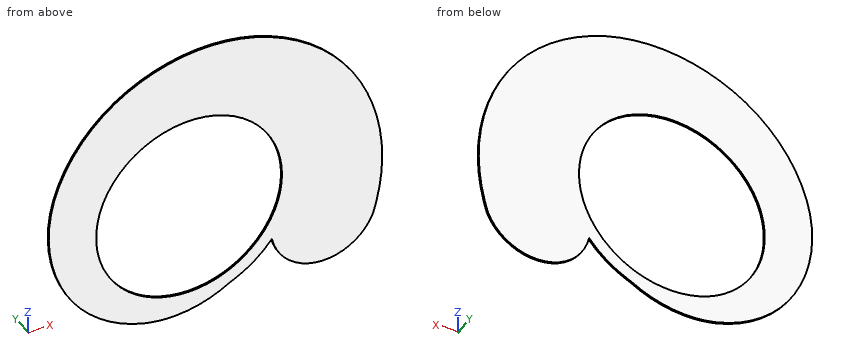
from build123d import *

# Parameters (mm, degrees)
F1_DEPTH = 3.175


with BuildPart() as f1:
    # F0 (on Front) → F1 (new body)
    with BuildSketch(Plane.XZ):
        with BuildLine():
            ThreePointArc((164.2657808805, 68.0411142745), (174.3836228557, 34.6870592545), (177.8, 0))
            ThreePointArc((177.8, 0), (174.3836228557, -34.6870592545), (164.2657808805, -68.0411142745))
            ThreePointArc((164.2657808805, -68.0411142745), (277.9531181005, -7.2739665138), (359.7319413837, -106.9217510028))
            ThreePointArc((359.7319413837, -106.9217510028), (359.3761364248, -115.4172186461), (358.3112136183, -123.8531837399))
            ThreePointArc((358.3112136183, -123.8531837399), (367.281161492, 8.8480312827), (328.531561761, 136.082228549))
            Line((328.531561761, 136.082228549), (164.2657808805, 68.0411142745))
        make_face()
        with BuildLine():
            ThreePointArc((68.0411142745, 164.2657808805), (125.723585695, 125.723585695), (164.2657808805, 68.0411142745))
            Line((164.2657808805, 68.0411142745), (328.531561761, 136.082228549))
            ThreePointArc((328.531561761, 136.082228549), (244.3258111618, 240.7675034736), (126.362069367, 305.0650216352))
            Line((126.362069367, 305.0650216352), (68.0411142745, 164.2657808805))
        make_face()
        with BuildLine():
            ThreePointArc((158.5532229762, -127.0870390081), (157.0041232469, -97.1378663495), (164.2657808805, -68.0411142745))
            ThreePointArc((164.2657808805, -68.0411142745), (137.7338592366, -112.4376450296), (99.5472631467, -147.32))
            ThreePointArc((99.5472631467, -147.32), (93.3013149914, -167.2172179653), (83.1243863135, -185.42))
            ThreePointArc((83.1243863135, -185.42), (124.3088906415, -160.740597571), (158.5532229762, -127.0870390081))
        make_face()
        with BuildLine():
            ThreePointArc((359.7319413837, -106.9217510028), (277.9531181005, -7.2739665138), (164.2657808805, -68.0411142745))
            Line((164.2657808805, -68.0411142745), (258.1319413837, -106.9217510028))
            Line((258.1319413837, -106.9217510028), (351.9981018868, -145.8023877311))
            ThreePointArc((351.9981018868, -145.8023877311), (355.3248382646, -134.8767336877), (358.3112136183, -123.8531837399))
            ThreePointArc((358.3112136183, -123.8531837399), (359.3761364248, -115.4172186461), (359.7319413837, -106.9217510028))
        make_face()
        with BuildLine():
            Line((258.1319413837, -106.9217510028), (164.2657808805, -68.0411142745))
            ThreePointArc((164.2657808805, -68.0411142745), (157.0041232469, -97.1378663495), (158.5532229762, -127.0870390081))
            ThreePointArc((158.5532229762, -127.0870390081), (248.3480567304, -208.0495691395), (351.9981018868, -145.8023877311))
            Line((351.9981018868, -145.8023877311), (258.1319413837, -106.9217510028))
        make_face()
        with BuildLine():
            ThreePointArc((-68.0411142745, 164.2657808805), (0, 177.8), (68.0411142745, 164.2657808805))
            Line((68.0411142745, 164.2657808805), (126.362069367, 305.0650216352))
            ThreePointArc((126.362069367, 305.0650216352), (2.514428483, 317.6217641107), (-116.6419101849, 281.5984815094))
            Line((-116.6419101849, 281.5984815094), (-68.0411142745, 164.2657808805))
        make_face()
        with BuildLine():
            ThreePointArc((83.1243863135, -185.42), (93.3013149914, -167.2172179653), (99.5472631467, -147.32))
            ThreePointArc((99.5472631467, -147.32), (84.2214695555, -156.5873049322), (68.0411142745, -164.2657808805))
            Line((68.0411142745, -164.2657808805), (77.7612734566, -187.7323210063))
            ThreePointArc((77.7612734566, -187.7323210063), (80.4511378852, -186.5954297752), (83.1243863135, -185.42))
        make_face()
        with BuildLine():
            ThreePointArc((-164.2657808805, 68.0411142745), (-125.723585695, 125.723585695), (-68.0411142745, 164.2657808805))
            Line((-68.0411142745, 164.2657808805), (-116.6419101849, 281.5984815094))
            ThreePointArc((-116.6419101849, 281.5984815094), (-204.8629851326, 208.4159123673), (-258.1319413837, 106.9217510028))
            Line((-258.1319413837, 106.9217510028), (-164.2657808805, 68.0411142745))
        make_face()
        with BuildLine():
            ThreePointArc((-164.2657808805, -68.0411142745), (-177.8, 0), (-164.2657808805, 68.0411142745))
            Line((-164.2657808805, 68.0411142745), (-258.1319413837, 106.9217510028))
            ThreePointArc((-258.1319413837, 106.9217510028), (-266.8448532831, 2.5095343628), (-234.6654012579, -97.2015918207))
            Line((-234.6654012579, -97.2015918207), (-164.2657808805, -68.0411142745))
        make_face()
        with BuildLine():
            ThreePointArc((-99.5472631467, -147.32), (-137.7338592366, -112.4376450296), (-164.2657808805, -68.0411142745))
            Line((-164.2657808805, -68.0411142745), (-234.6654012579, -97.2015918207))
            ThreePointArc((-234.6654012579, -97.2015918207), (-172.5099209033, -168.9661068295), (-87.4814326387, -211.1988611321))
            Line((-87.4814326387, -211.1988611321), (-79.0449703485, -190.8314394527))
            ThreePointArc((-79.0449703485, -190.8314394527), (-91.908148752, -170.3064913493), (-99.5472631467, -147.32))
        make_face()
        with BuildLine():
            Line((77.7612734566, -187.7323210063), (68.0411142745, -164.2657808805))
            ThreePointArc((68.0411142745, -164.2657808805), (34.6870592545, -174.3836228557), (0, -177.8))
            ThreePointArc((0, -177.8), (-34.6870592545, -174.3836228557), (-68.0411142745, -164.2657808805))
            Line((-68.0411142745, -164.2657808805), (-79.0449703485, -190.8314394527))
            ThreePointArc((-79.0449703485, -190.8314394527), (-63.7096435601, -206.143169746), (-45.4758683551, -217.8543086339))
            ThreePointArc((-45.4758683551, -217.8543086339), (18.4051257388, -212.0494957439), (77.7612734566, -187.7323210063))
        make_face()
        with BuildLine():
            ThreePointArc((-68.0411142745, -164.2657808805), (-84.2214695555, -156.5873049322), (-99.5472631467, -147.32))
            ThreePointArc((-99.5472631467, -147.32), (-91.908148752, -170.3064913493), (-79.0449703485, -190.8314394527))
            Line((-79.0449703485, -190.8314394527), (-68.0411142745, -164.2657808805))
        make_face()
        with BuildLine():
            ThreePointArc((-87.4814326387, -211.1988611321), (-66.6429296743, -215.563425688), (-45.4758683551, -217.8543086339))
            ThreePointArc((-45.4758683551, -217.8543086339), (-63.7096435601, -206.143169746), (-79.0449703485, -190.8314394527))
            Line((-79.0449703485, -190.8314394527), (-87.4814326387, -211.1988611321))
        make_face()
    extrude(amount=F1_DEPTH)


solid = f1.part
Could you check a few things on this model? Use its own coordinates, in mm. Give positions to 0.01 mm unless a question says otherwise; leave off trailing zeros. Order: outer loops, then holes, each group sorted by start corner. A loop starts at its lowest first (then second) coordinate and runs counter-clockwise, first axis right, second up.
Item 1: If we section it at C-C, the plane x = -31: Write out the boundary of the cut face in (y, z) (3 decimals), plus the area to 4 significant figures.
Item 2: I'm going to push flat-ended pins straight in: pin 1 (1.5 mm diameter, centred on y = -2, z = 188.5, fed in from +X); pin 2 (8 mm diameter, centred on x = -55.5, z = 162, fed in from +Y); pin 3 (1 mm diameter, centred on x = -149.5, y = -2, fed in from -Z). Where does each tip first touch, or does it pass through?
Item 3: I need wall thicknesses on line 1 (X direction, y = -2, z = 11); line 2 (X direction, y = -0.8, z = 58.5); line 3 (X direction, y = -2.6, z = -152). Which ranges of each line are inside material? Lowest first, please.
Item 4: If we section it at D-D, the plane z = 230: Write out the boundary of the cut face in (x, y) (3 decimals).
Item 5: If we section it at A-A, the plane z = -87.5: Write out the boundary of the cut face in (x, y) (3 decimals), plus the area to 3 significant figures.
Item 6: If we section it at B-B, the plane y = -1.8: Write out the boundary of the cut face in (x, z), plus the area to 3 significant figures.
Values:
1. outline: (-3.175, -218.215) - (0, -218.215) - (0, -175.077) - (-3.175, -175.077) - close; (-3.175, 175.077) - (0, 175.077) - (0, 312.568) - (-3.175, 312.568) - close
1. area: 573.5 mm2
2. pin 1: stops at x = 295.43
2. pin 2: passes through
2. pin 3: stops at z = -185.05
3. line 1: x = -267.68 to -177.46, 177.46 to 367.03
3. line 2: x = -267.37 to -167.9, 167.9 to 358.11
3. line 3: x = -192.14 to -92.24, 92.24 to 134.86, 167.08 to 349.18
4. outline: (-185.53, -3.175) - (256.602, -3.175) - (256.602, 0) - (-185.53, 0) - close
5. outline: (-239.831, -3.175) - (-154.779, -3.175) - (-154.779, 0) - (-239.831, 0) - close; (154.779, -3.175) - (365.631, -3.175) - (365.631, 0) - (154.779, 0) - close
5. area: 939 mm2
6. outline: (-258.13, 106.92) arc R266.7 ccw to (-234.67, -97.2) arc R241.3 ccw to (-87.48, -211.2) arc R215.9 ccw to (77.76, -187.73) arc R203.2 ccw to (158.55, -127.09) arc R101.6 ccw to (352, -145.8) arc R368.3 ccw to (328.53, 136.08) arc R342.9 ccw to (126.36, 305.07) arc R317.5 ccw to (-116.64, 281.6) arc R292.1 ccw to start; hole circle Ø355.6 at (0, 0)
6. area: 174,000 mm2
